Design review of the part built by this model. Coordinates are the model's own, in mm. Face numbers are marked on the shaded views. Round coordinates to 2 decimals unless told otherwise and drop trailing zeros. Write each loop counter-clockwise with the first axis right and the second up, starting at its lowest first coordinate (ties: lowest second). Pieces come first, ordered by that corner, then holes. Notation, with made-up numbers: M 71.5,-22 L 95.5,-22 A9 ccw 95.5,-7 Z; hole C -5.75,-37.5 d11. An arc over 180 degrees is marked long. One line per question, with ' | ' between items. Start each with the question number.
Item 1: Draft analysis for pull direction Y (two halves, no side actions). For the marked faces 1, 2, 3 and 4, state which applies: released by +Y, released by -Y, zero draft, split by the parting line, or undercut.
Item 2: Add section B-B, the plane z = 19.5. State the section outline as (x, y) points.
Item 3: For L1, parallel to Z at x = 2, y = -12; L2, parallel to Y at x = 21.5, z = 3.5; L3, parallel to Y at x = -6, z = 1.25, list the stretches that pass through material, from the lowest coordinate up.
Item 4: Add section A-A, the plane y = -34.5. State the section outline as (x, z) points.
Item 5: Add section C-C, the plane y = -7. State the section outline as (x, z) points.
```python
from build123d import *

# Parameters (mm, degrees)
F0_W     = 95.25
F0_H     = 60.3318884472
F1_DEPTH = 25.4
F3_DEPTH = 95.25
F5_DEPTH = 95.25
F6_R     = 8.5166000229
F7_DEPTH = 2.54


with BuildPart() as f1:
    # F0 (on Top) → F1 (new body)
    with BuildSketch(Plane.XY):
        with Locations((6.9396421313, -14.7977671586)):
            Rectangle(F0_W, F0_H)
    extrude(amount=F1_DEPTH)

    # F2 (on face) → F3 (cut)
    with BuildSketch(Plane.YZ.offset(54.5646421313)):
        with BuildLine():
            Line((-17.5997193688, 3.2119287359), (-20.3140247613, 0))
            Line((-20.3140247613, 0), (-14.7977671586, 0))
            Line((-14.7977671586, 0), (-9.2815095559, 0))
            Line((-9.2815095559, 0), (-11.9958061003, 3.2119362131))
            add(Edge.make_bspline(
                [(-17.5997193688, 3.2119287359), (-15.7335996163, 4.4085908758), (-15.1440525404, 5.4683826364), (-13.1693625568, 4.4868656847), (-11.9958061003, 3.2119362131)],
                knots=[0, 0, 0, 0, 0.4999998654, 1, 1, 1, 1], degree=3))
        make_face()
    extrude(amount=-F3_DEPTH, mode=Mode.SUBTRACT)

    # F4 (on face) → F5 (cut)
    with BuildSketch(Plane(origin=(0, 15.368177065, 0), x_dir=(-1, 0, 0), z_dir=(0, 1, 0))):
        Polygon((-60.7218779624, 31.5345525742), (-58.8849112391, 0), (-23.1661610305, 31.5345525742), align=None)
    extrude(amount=-F5_DEPTH, mode=Mode.SUBTRACT)

    # F6 (on face) → F7 (cut)
    with BuildSketch(Plane(origin=(25.7930277101, 0, 29.2154046497), x_dir=(0.7496503208, 0, -0.6618341156), z_dir=(0.6618341156, 0, 0.7496503208))):
        with Locations((25.0689592212, -14.590062201)):
            Circle(F6_R)
    extrude(amount=-F7_DEPTH, mode=Mode.SUBTRACT)


solid = f1.part
```
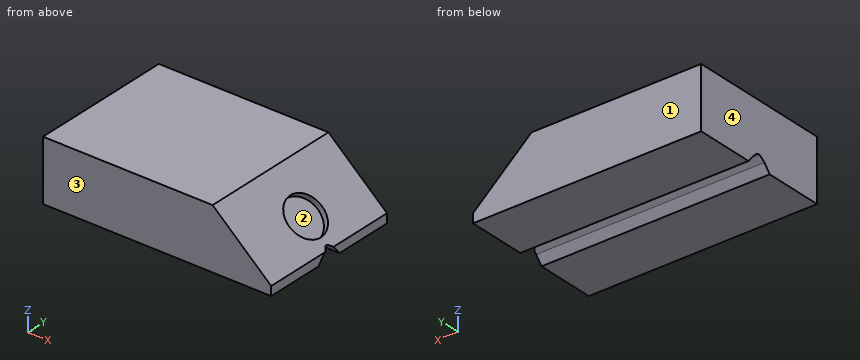
Computed values:
1) face 1: released by +Y | face 2: undercut | face 3: released by -Y | face 4: zero draft
2) outline: M -40.69,-44.96 L 36.8,-44.96 L 36.8,15.37 L -40.69,15.37 Z
3) L1: z = 3.22 to 25.4 | L2: y = -44.96 to -17.16, -12.27 to 15.37 | L3: y = -44.96 to -19.26, -10.34 to 15.37
4) outline: M -40.69,0 L 54.56,0 L 54.56,3.81 L 30.11,25.4 L -40.69,25.4 Z
5) outline: M -40.69,0 L 54.56,0 L 54.56,3.81 L 47.48,10.07 L 45.8,8.16 L 40.01,13.28 L 41.69,15.18 L 30.11,25.4 L -40.69,25.4 Z
